Model file for the job. Use its own axes, mm. Face numbers are marked on the shaded views. A direction names the side the tool comes from. Round coordinates to 2 decimals unless told otherwise and drop trailing zeros. Order: outer loops, then holes, each group sorted by start corner. A loop starts at its lowest first (then second) coordinate and runs counter-clockwise, first axis right, second up. Notation, with made-up numbers: (85.5, -29) - (125.5, -29) arc R19 ccw to (125.5, -7) - close; hole circle Ø1 at (-16, 9.25). An arc over 180 degrees is marked (long way). Put each result on its own line as item: value. Start each with the question number.
Item 1: Saw through at B-B on z = -9. State how many separate pieces and enclosed holes the cut face has, plus the area to 3 significant figures.
Item 2: Saw through at A-A on y = 20. List the corners of the cut face in (x, z), plus the area to 3 significant figures.
Item 3: Probe probe 1 along X at (y, z) = (11, -10); probe 2 along X at (y, z) = (26.5, -2.5); probe 3 along Z at (x, y) = (28, 11.5). List the from-to ranges inside material, lowest first.
Item 4: Saw through at C-C on x = -7. List the corners of the cut face in (y, z).
Item 5: Pin check, flat tips, straight feed: pin 1 Ø20 at (x, y) = (12.5, 24) entering from -Z; pin 2 Ø1.5 at (x, y) = (56.5, 16.5) entering from -Z; pin 3 Ø6 at (y, z) = (16.5, -12) entering from -X. Stop position of each tip, or through.
Item 6: Which spindle directions (+Z, -Z, +X, -X, +Y, -Y) get a long thin tool onto all of the face, cutting with end or side? Do the marked faces 1 and 2. Say none if no direction does.
Item 7: Mould opens along Y. For the marked faces 3, 4, 5 and 6 say: pulls with the +Y half, pulls with the -Y half, needs draft (parallel to the pull), parting line crosses it, or undercut.
```python
from build123d import *

# Parameters (mm, degrees)
BOSS_EXTRUDE1_DEPTH = 40
SKETCH2_R           = 13
CUT_EXTRUDE1_DEPTH  = 210.771304043
CHAMFER1_SIZE       = 5
FILLET3_R           = 2
CHAMFER2_SIZE       = 2


with BuildPart() as part:
    # Sketch1 → Boss-Extrude1 (new body)
    with BuildSketch(Plane(origin=(0, 0, 0), x_dir=(1, 0, 0), z_dir=(0, 1, 0))):
        Polygon((41, 0), (-41, 0), (-41, 20), (-49.25, 20), (-49.25, 0), (-52.4, 0), (-52.4, 20), (-101, 20), (-101, -40), (101, -40), (101, 20), (52.4, 20), (52.4, 0), (49.25, 0), (49.25, 20), (41, 20), align=None)
    extrude(amount=BOSS_EXTRUDE1_DEPTH)

    # Sketch2 → Cut-Extrude1 (cut, through all)
    with BuildSketch(Plane.ZY.offset(101)):
        with Locations((-20, 20)):
            Circle(SKETCH2_R)
    extrude(amount=-CUT_EXTRUDE1_DEPTH, mode=Mode.SUBTRACT)

    # Chamfer1
    chamfer1_edges = [part.edges().sort_by_distance(p)[0] for p in [
        (-41, 20, 0),
        (41, 20, 0),
    ]]
    chamfer(chamfer1_edges, length=CHAMFER1_SIZE)

    # Fillet3
    fillet3_edges = [part.edges().sort_by_distance(p)[0] for p in [
        (41, 36.5, -20),
        (49.25, 36.5, -20),
        (52.4, 36.5, -20),
        (-52.4, 36.5, -20),
        (-49.25, 36.5, -20),
        (-41, 36.5, -20),
        (41, 3.5, -20),
        (49.25, 3.5, -20),
        (52.4, 3.5, -20),
        (-52.4, 3.5, -20),
        (-49.25, 3.5, -20),
        (-41, 3.5, -20),
        (-36, 20, 0),
        (36, 20, 0),
        (41, 20, -5),
        (-41, 20, -5),
    ]]
    fillet(fillet3_edges, radius=FILLET3_R)

    # Chamfer2
    chamfer2_edges = [part.edges().sort_by_distance(p)[0] for p in [
        (49.25, 20, 0),
        (-49.25, 20, 0),
    ]]
    chamfer(chamfer2_edges, length=CHAMFER2_SIZE)


solid = part.part
```
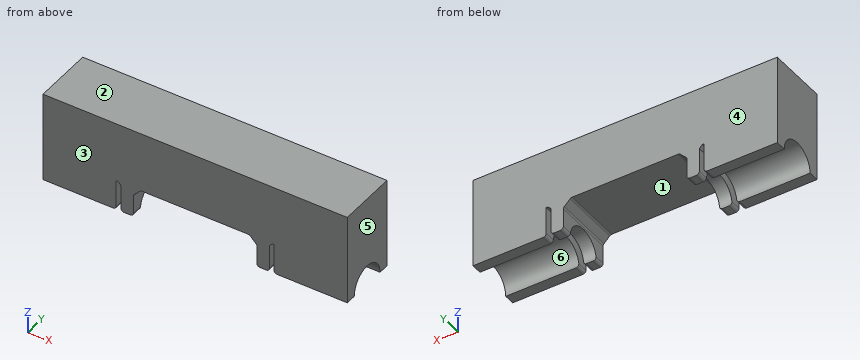
Results found:
1. separate pieces: 8
1. enclosed holes: 0
1. area: 2,970 mm²
2. outline: (-101, -7) - (-52.4, -7) - (-52.4, 0) - (-51.25, 0) - (-49.25, -2) - (-49.25, -7) - (-41, -7) - (-41, -5.83) arc R2 cw to (-40.41, -4.41) - (-36.59, -0.59) arc R2 cw to (-35.17, 0) - (35.17, 0) arc R2 cw to (36.59, -0.59) - (40.41, -4.41) arc R2 cw to (41, -5.83) - (41, -7) - (49.25, -7) - (49.25, -2) - (51.25, 0) - (52.4, 0) - (52.4, -7) - (101, -7) - (101, 40) - (-101, 40) - close
2. area: 8,910 mm²
3. probe 1: x = -101 to -52.4, -49.25 to -41, 41 to 49.25, 52.4 to 101
3. probe 2: x = -101 to -52.4, -49.25 to -38.5, 38.5 to 49.25, 52.4 to 101
3. probe 3: z = 0 to 40
4. outline: (0, 0) - (40, 0) - (40, 40) - (0, 40) - close
5. pin 1: stops at z = 0
5. pin 2: stops at z = -7.71
5. pin 3: passes through
6. face 1: -Z, +Y, -Y
6. face 2: +Z, +X, -X, +Y, -Y
7. face 3: pulls with the -Y half
7. face 4: pulls with the +Y half
7. face 5: needs draft
7. face 6: undercut
